Design review of the part built by this model. Coordinates are the model's own, in mm. Face numbers are marked on the shaded views. A direction names the side the tool comes from. Coordinates: 2 decimals unless noted, no trailing zeros. Loops run counter-clockwise (first coordinate to the right, second up) from the corner with the lowest first, then second, coordinate; pieces in that order, holes last. Notation, with made-up numbers: M 35.5,52.5 L 39.5,52.5 A11 ccw 39.5,69.5 Z; hole C 9,59 d6. An arc over 180 degrees is marked long. One line per item, written item: value.
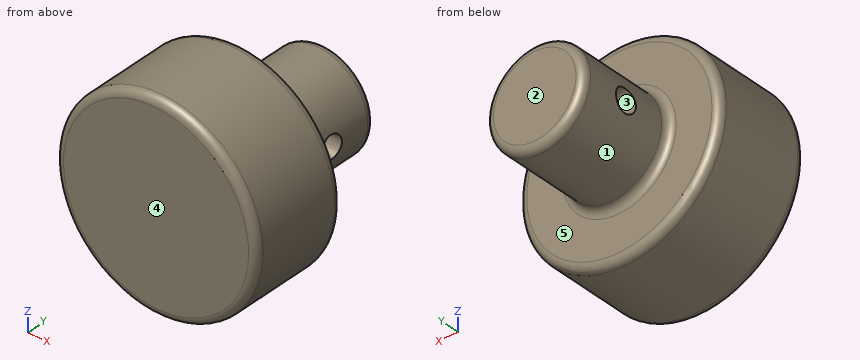
```python
from build123d import *

# Parameters (mm, degrees)
SKETCH2_R               = 6.5
BOSS_EXTRUDE1_DEPTH     = 6.35
SKETCH3_R               = 3.175
BOSS_EXTRUDE2_DEPTH     = 6.35
CUT_EXTRUDE1_DEPTH      = 6.35
CUT_EXTRUDE1_DEPTH_BACK = 6.35
SKETCH4_R               = 0.75
FILLET1_R               = 0.5


with BuildPart() as part:
    # Sketch2 → Boss-Extrude1 (new body)
    with BuildSketch(Plane(origin=(0, 0, 0), x_dir=(1, 0, 0), z_dir=(0, 1, 0))):
        with Locations(Location((0, 0, 0), (0, 0, 270))):
            Circle(SKETCH2_R)
    extrude(amount=BOSS_EXTRUDE1_DEPTH)

    # Sketch3 → Boss-Extrude2 (add)
    with BuildSketch(Plane(origin=(0, 6.35, 0), x_dir=(1, 0, 0), z_dir=(0, 1, 0))):
        with Locations(Location((0, 0, 0), (0, 0, 270))):
            Circle(SKETCH3_R)
    extrude(amount=BOSS_EXTRUDE2_DEPTH)

    # Sketch4 → Cut-Extrude1 (cut, two sides: drawn at the far end of the back side and taken through both)
    with BuildSketch(Plane(origin=(0, 0, 0), x_dir=(0, 0, -1), z_dir=(1, 0, 0)).offset(-CUT_EXTRUDE1_DEPTH_BACK)):
        with Locations(Location((0, 9.525, 0), (0, 0, 180))):
            Circle(SKETCH4_R)
    extrude(amount=CUT_EXTRUDE1_DEPTH + CUT_EXTRUDE1_DEPTH_BACK, mode=Mode.SUBTRACT)

    # Fillet1
    fillet1_edges = [part.edges().sort_by_distance(p)[0] for p in [
        (0, 0, -6.5),
        (0, 6.35, -6.5),
        (0, 6.35, -3.175),
        (0, 12.7, -3.175),
    ]]
    fillet(fillet1_edges, radius=FILLET1_R)


solid = part.part
```
(1) To check wall thickness, follow line 1 along Y through (x, z) = (-0.25, 0) (3 decimals); line 2 along Y through (x, z) = (-0.5, 5.5); line 3 along X through (y, z) = (5.5, -0.25). State the ranges of each line that lie inside material, in increasing order. Write a range as [from, to].
Reply:
line 1: y = [0, 8.775], [10.275, 12.7]
line 2: y = [0, 6.35]
line 3: x = [-6.5, 6.5]
(2) We need section A-A on z = 0. State the section outline as (x, y) points (3 decimals).
Reply:
outline: M -6.5,0.5 A0.5 ccw -6,0 L 6,0 A0.5 ccw 6.5,0.5 L 6.5,5.85 A0.5 ccw 6,6.35 L 3.675,6.35 A0.5 cw 3.175,6.85 L 3.175,8.775 L -3.175,8.775 L -3.175,6.85 A0.5 cw -3.675,6.35 L -6,6.35 A0.5 ccw -6.5,5.85 Z; M -3.175,10.275 L 3.175,10.275 L 3.175,12.2 A0.5 ccw 2.675,12.7 L -2.675,12.7 A0.5 ccw -3.175,12.2 Z
(3) Tool access review of the marked faces 4 and 5: name each direction out of +Z, -Z, +X, -X, +Y, -Y from which nothing blocks a thin tool from reaching the whole face with its end or side.
Reply:
face 4: +Z, -Z, +X, -X, -Y
face 5: +Y
(4) We need section C-C on x = 0. State the section outline as (y, z) points (3 decimals), then the cut area to 3 significant figures.
Reply:
outline: M 0,-6 A0.5 ccw 0.5,-6.5 L 5.85,-6.5 A0.5 ccw 6.35,-6 L 6.35,-3.675 A0.5 cw 6.85,-3.175 L 12.2,-3.175 A0.5 ccw 12.7,-2.675 L 12.7,2.675 A0.5 ccw 12.2,3.175 L 6.85,3.175 A0.5 cw 6.35,3.675 L 6.35,6 A0.5 ccw 5.85,6.5 L 0.5,6.5 A0.5 ccw 0,6 Z; hole C 9.525,0 d1.5
area: 121 mm2
(5) Mouldability with a two-part tool opening along Z and no side actions: class the marked faces 1, 2 and 3 as released by +Z, released by -Z, zero draft, split by the parting line, or undercut.
Reply:
face 1: split by the parting line
face 2: zero draft
face 3: undercut
(6) Insertion check: pin 1 (2 mm diameter, centred on y = 2, z = -3, fed in from -X); pin 2 (4 mm diameter, centred on y = 9.5, z = 2.5, fed in from +X). Each pin has a flat end and moves straight along its axis. Give the tip position at first contact, or say it passes through.
Reply:
pin 1: stops at x = -6.18
pin 2: stops at x = 3.13
(7) We need section B-B on y = 2.5. State the section outline as (x, z) points, then the cut area to 3 significant figures.
Reply:
outline: C 0,0 d13
area: 133 mm2
